Geometry check sheet. Reference: drawing and pictorial views, mm from the part's lowest x, y, z. A direction names the side the tool comes from. Give positions to 0.01 mm unless a question says otherwise; leave off trailing zeros. Order: outer loops, then holes, each group sorted by start corner. A loop starts at its lowest first (then second) coordinate and runs counter-clockwise, first axis right, second up.
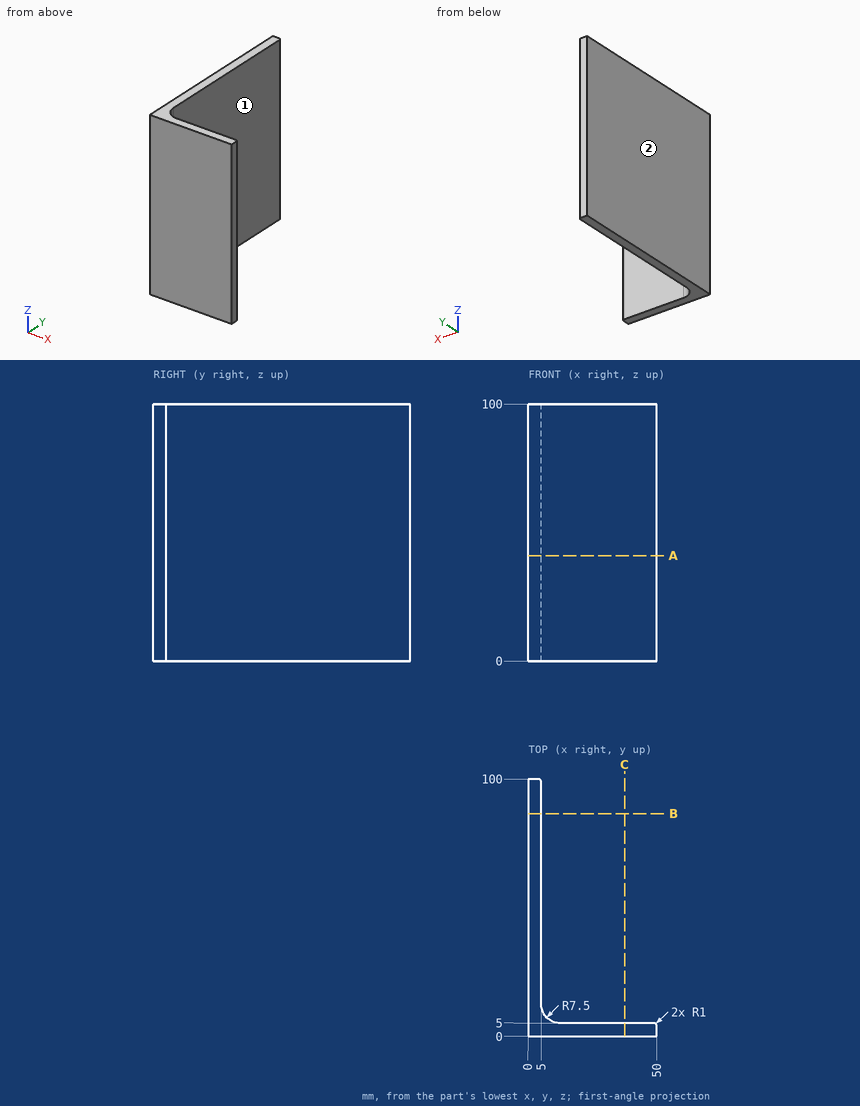
(1) Cross-section at B-B on y = 86.5. Enter the section's corners in (x, z), then the cut area to 3 significant figures.
Response values:
outline: (0, 0) - (5, 0) - (5, 100) - (0, 100) - close
area: 500 mm2
(2) Set-up check for the marked faces 1 and 2: record each of +Z, -Z, +X, -X, +Y, -Y from which the full face is reachable in a straight line by a thin tool's end or side.
Response values:
face 1: +Z, -Z, +X, +Y
face 2: +Z, -Z, -X, +Y, -Y
(3) Gauge pin test, flat ends, axial feed: pin 1 Ø4 at (x, z) = (27.5, 22) entering from +Y; pin 2 Ø3 at (y, z) = (84.5, 35.5) entering from +X; pin 3 Ø4 at (y, z) = (12, 13.5) entering from +X. Record the tip position at first contact, or that the pin passes through.
Response values:
pin 1: stops at y = 5
pin 2: stops at x = 5
pin 3: stops at x = 5.43
(4) Cross-section at A-A on z = 41. Enter the section's corners in (x, y), then the cut area to 3 significant figures.
Response values:
outline: (0, 0) - (50, 0) - (50, 4) arc R1 ccw to (49, 5) - (12.5, 5) arc R7.5 cw to (5, 12.5) - (5, 99) arc R1 ccw to (4, 100) - (0, 100) - close
area: 737 mm2
(5) Material ranges on L1, parallel to Y at x = 36, z = 39; L2, parallel to Y at x = 10, z = 80, recorded low to high.
Response values:
L1: y = 0 to 5
L2: y = 0 to 5.43
